Input: part model. Units: mm. Frame: model coordinates. A direction names the side the tool comes from. Coordinates: 2 decimals unless noted, no trailing zeros. Order: outer loops, then holes, each group sorted by start corner. A loop starts at its lowest first (then second) coordinate and runs counter-clockwise, first axis right, second up. Notation, with made-up numbers: M 19,78.25 L 26,78.25 A18 ccw 26,109.25 Z; hole C 32.25,40 d11. An arc over 180 degrees is marked long. One line per item, written item: value.
```python
from build123d import *

# Parameters (mm, degrees)
F0_W     = 38.1
F0_H     = 31.75
F1_DEPTH = 25.4
F3_DEPTH = 25.4


with BuildPart() as f1:
    # F0 (on Front) → F1 (new body)
    with BuildSketch(Plane.XZ):
        with Locations((19.05, 15.875)):
            Rectangle(F0_W, F0_H)
    extrude(amount=-F1_DEPTH)

    # F2 (on face) → F3 (cut)
    with BuildSketch(Plane.XZ):
        Polygon((25.4, 12.93213), (38.1, 12.93213), (38.1, 31.75), (12.7, 31.75), align=None)
    extrude(amount=-F3_DEPTH, mode=Mode.SUBTRACT)


solid = f1.part
```
(1) Cut plane B-B on x = 30. Output: boundary loops of the cut face in (y, z), plus the area to 3 significant figures.
Data:
outline: M 0,0 L 25.4,0 L 25.4,12.93 L 0,12.93 Z
area: 328 mm2
(2) Ray query, line 1 (Z direction, x = 26.5, y = 10.25); line 2 (Z direction, x = 24, y = 18.25); line 3 (X direction, y = 20.75, z = 17). Return the intervals inside material, ascending. Write a range as from..to.
Data:
line 1: z = 0..12.93
line 2: z = 0..15.01
line 3: x = 0..22.65
(3) First-contact query: pin 1 (1 mm diameter, centred on y = 6.5, z = 23.5, fed in from +X); pin 2 (8 mm diameter, centred on y = 11.5, z = 27.5, fed in from +X); pin 3 (6.5 mm diameter, centred on x = 33.5, y = 6.5, fed in from +Z); pin 4 (5 mm diameter, centred on x = 20.5, z = 27.5, fed in from -Y). Flat tips, straight axial feed; report the tip coordinate or a pass-through.
Data:
pin 1: stops at x = 18.61
pin 2: stops at x = 18.27
pin 3: stops at z = 12.93
pin 4: passes through
(4) Cut plane C-C on z = 29. Output: boundary loops of the cut face in (x, y).
Data:
outline: M 0,0 L 14.56,0 L 14.56,25.4 L 0,25.4 Z
(5) Cut plane A-A on y = 2.75. Output: boundary loops of the cut face in (x, z), plus the area to 3 significant figures.
Data:
outline: M 0,0 L 38.1,0 L 38.1,12.93 L 25.4,12.93 L 12.7,31.75 L 0,31.75 Z
area: 851 mm2
(6) Access query for faces 1 (the flat face through (0, 13, 16)), 2 (the flat face through (32, 13, 12.932)). Directions: +Z, -Z, +X, -X, +Y, -Y. A direction counts if a zero-diameter tool reaches every point of the face in a straight line with its end or side. Return the directions, or none.
Data:
face 1: +Z, -Z, -X, +Y, -Y
face 2: +Z, +X, +Y, -Y
